Model file for the job. Use its own axes, mm. A direction names the side the tool comes from. Round coordinates to 2 decimals unless told otherwise and drop trailing zeros. Order: outer loops, then holes, each group sorted by start corner. A loop starts at its lowest first (then second) coordinate and runs counter-clockwise, first axis right, second up. Notation, with made-up numbers: M -35.5,76.5 L 2.5,76.5 A31 cw 2.5,109.5 Z; hole C -11.75,23.5 d10. An arc over 180 degrees is marked long. Return JSON: item names as keys, results as strings. Group by question number.
Item 1: Slice it at A-A on z = 2. Give the number of separate pieces and of enclosed holes in the cut face, then the cut area to 3 significant figures.
Item 2: Which spindle directions (+Z, -Z, +X, -X, +Y, -Y) get a long thin tool onto all of the face, cutting with end or side? Do faces 4 (the face through (-17, 3, 2)), 5 (the face through (-6.25, -6, 0)), 6 (the face through (0, 12, 1)), 7 (the face through (-0.1, -9.2, -2)), 8 (the face through (11, -1, 4)). Say none if no direction does.
Item 3: Slice it at B-B on z = -0.5. Write the cut outline in (x, y) (3 decimals), then the cut area to 3 significant figures.
Item 4: Pin check, flat tips, straight feed: pin 1 Ø1.6 at (x, z) = (-17, 1.5) entering from +Y; pin 2 Ø2.5 at (x, y) = (-12, 0) entering from +Z; pin 3 Ø5 at (x, z) = (-3, 0) entering from +Y; pin 4 Ø2.5 at (x, y) = (0, 16) entering from -Z. Stop position of each tip, or through.
Item 5: Probe line 1 along Y through (x, z) = (0, 2) (3 decimals); line 2 along X through (y, z) = (14, 3.25); line 3 along X through (y, z) = (3, 4.5). List the from-to ranges inside material, lowest first.
Item 6: Pull direction X, two halves, no side cores. Call faces 1 (the face through (17, 3, 2)), 2 (the face through (0, 18, 2)), 3 (the face through (-8, -8, 1)): pulls with the +X half, pulls with the -X half, needs draft (parallel to the pull), parting line crosses it, or undercut.
Autodesk Inventor part; units mm, degrees
ref_plane "YZ Plane" through (0, 0, 0) normal (1, 0, 0) x (0, 1, 0)
ref_plane "XZ Plane" through (0, 0, 0) normal (0, 1, 0) x (-1, 0, 0)
ref_plane "XY Plane" through (0, 0, 0) normal (0, 0, 1) x (1, 0, 0)
sketch "Sketch1" plane through (0, 0, 0) normal (0, 0, 1) x (1, 0, 0)
  circle A0 centre (0, 0) radius 18
  line L0 (0, 0) -> (0, 18) construction
  line L1 (4, 17.5499) -> (4, 11.9999)
  line L2 (4, 11.9999) -> (8.5659, 15.8312)
  line L3 (0, 0) -> (18, 0) construction
  line L4 (-4, 17.5499) -> (-4, 11.9999)
  line L5 (-4, 11.9999) -> (-8.5659, 15.8312)
  line L6 (4, -17.5499) -> (4, -11.9999)
  line L7 (4, -11.9999) -> (8.5659, -15.8312)
  line L8 (-4, -11.9999) -> (-8.5659, -15.8312)
  line L9 (-4, -17.5499) -> (-4, -11.9999)
  dimension "d1" = 50
  dimension "d2" = 36
  dimension "d3" = 5.55
  dimension "d4" = 8
extrude "Extrusion1" add sketch "Sketch1" along normal blind 3.5
sketch "Sketch2" plane through (0, 0, 0) normal (0, 1, 0) x (-1, 0, 0)
  line L0 (0, 0) -> (0, 6)
  line L1 (0, 6) -> (-3.5, 6)
  line L2 (-3.5, 6) -> (-6.875, 3.5)
  line L3 (8.5659, 3.5) -> (-18, 3.5)
  line L4 (8.5659, 0) -> (8.5659, 0)
  line L5 (-6.875, 3.5) -> (0, 3.5)
  line L6 (-8.5659, 3.5) -> (-4, 3.5)
  point P0 (-18, 0)
  point P1 (18, 0)
  dimension "d7" = 3.5
  dimension "d8" = 6
  dimension "d9" = 13.75
revolve "Revolution1" add sketch "Sketch2" angle 360 about axis through (0, 0, 0) along (0, 0, 1)
sketch "Sketch6" plane through (0, 0, 0) normal (1, 0, 0) x (0, 1, 0)
  circle A0 centre (-18, 0.2) radius 0.2
  line L0 (18, 0) -> (-18, 0)
  line L1 (-18, 0) -> (-18, 3.5)
  line L2 (0, 0) -> (0, 9.8131)
  point P0 (-18, 0.4)
  dimension "d28" = 0.4
revolve "Revolution2" add sketch "Sketch6" angle 360 about axis through (0, 0, 0) along (0, 0, 1) picked at (-18.0623, 0.1764) contours A0 L1
sketch "Sketch7" plane through (0, 0, 3.5) normal (0, 0, 1) x (1, 0, 0)
  line L0 (4, 17.5499) -> (4, 11.9999)
  line L1 (4, 11.9999) -> (8.5659, 15.8312)
  line L2 (-4, 17.5499) -> (-4, 11.9999)
  line L3 (-4, 11.9999) -> (-8.5659, 15.8312)
  line L4 (-4, -11.9999) -> (-8.5659, -15.8312)
  line L5 (-4, -17.5499) -> (-4, -11.9999)
  line L6 (4, -17.5499) -> (4, -11.9999)
  line L7 (4, -11.9999) -> (8.5659, -15.8312)
  line L8 (4, -17.5499) -> (4, -18.3914)
  line L9 (8.5659, -15.8312) -> (9.2402, -16.397)
  line L10 (0, 0) -> (0, -19.1276)
  line L11 (0, 0) -> (-12.703, 0)
  circle A0 centre (0, 0) radius 18.8214
  line L12 (-4, -17.5499) -> (-4, -18.3914)
  line L13 (-8.5659, -15.8312) -> (-9.2402, -16.397)
  line L14 (4, 17.5499) -> (4, 18.3914)
  line L15 (8.5659, 15.8312) -> (9.2402, 16.397)
  line L16 (-4, 17.5499) -> (-4, 18.3914)
  line L17 (-8.5659, 15.8312) -> (-9.2402, 16.397)
extrude "Extrusion5" cut sketch "Sketch7" against normal through all contours L14 A0 L15 L1 L0 | L16 L2 L3 L17 A0 | A0 L8 L6 L7 L9 | L13 L4 L5 L12 A0
sketch "Sketch4" plane through (0, 0, 3.5) normal (0, 0, 1) x (1, 0, 0)
  line L0 (0, 0) -> (0, -18)
  arc A0 (-8.5659, 15.8312) -> (-8.5659, -15.8312) centre (0, 0) ccw
  line L1 (0, -8.925) -> (-6.25, -8.925)
  line L2 (-6.25, -8.925) -> (-6.25, -6.875)
  line L3 (-6.25, -6.875) -> (0, -6.875)
  circle A1 centre (0, 0) radius 6.875
  line L4 (0, -8.925) -> (6.25, -8.925)
  line L5 (6.25, -8.925) -> (6.25, -6.875)
  line L6 (6.25, -6.875) -> (0, -6.875)
  point P0 (-4, -17.5499)
  point P1 (4, -17.5499)
  dimension "d12" = 2.05
  dimension "d13" = 12.5
extrude "Extrusion2" cut sketch "Sketch4" against normal through all contours L6 L5 L4 L0 | L0 L1 L2 L3
sketch "Sketch3" plane through (0, 0, 0) normal (0, 0, -1) x (-1, 0, 0)
  line L0 (8.5659, -15.8312) -> (4, -11.9999)
  line L1 (8.5659, -15.8312) -> (4, -11.9999)
  line L2 (4, -11.9999) -> (8, -11.9999)
  line L3 (8, -11.9999) -> (8, -3.9)
  line L4 (8, -3.9) -> (-1.347, -3.9)
  line L5 (0, 0) -> (0, -22.6953) construction
  line L6 (8.5659, -15.8312) -> (9.347, -21.3508)
  line L7 (9.347, -21.3508) -> (0, -21.3508)
  line L8 (4, 11.9999) -> (8.5659, 15.8312)
  line L9 (8.5659, 15.8312) -> (4, 11.9999)
  line L10 (4, 11.9999) -> (-4, 11.9999)
  line L11 (-8.5659, 15.8312) -> (-4, 11.9999)
  line L12 (-4, 11.9999) -> (-8.5659, 15.8312)
  line L13 (-8.5659, 15.8312) -> (-8.5659, 22.0204)
  line L14 (-8.5659, 22.0204) -> (9.347, 21.5839)
  line L15 (9.347, 21.5839) -> (8.5659, 15.8312)
  line L16 (-8.5659, -15.8312) -> (-4, -11.9999)
  line L17 (-4, -11.9999) -> (-8, -11.9999)
  line L18 (-8, -11.9999) -> (-8, -3.9)
  line L19 (-8, -3.9) -> (-1.347, -3.9)
  line L20 (-8.5659, -15.8312) -> (-9.347, -21.3508)
  line L21 (-9.347, -21.3508) -> (0, -21.3508)
  line L22 (6.25, -8.925) -> (6.25, -6.875)
  line L23 (6.25, -7.9) -> (0, -7.9) construction
  line L24 (6.25, -7.9) -> (6.25, -5.4)
  line L25 (6.25, -5.4) -> (6.25, -3.9)
  dimension "d11" = 16
  dimension "d16" = 2.5
  dimension "d17" = 1.5
extrude "Extrusion3" cut sketch "Sketch3" against normal blind 1.5
sketch "Sketch5" plane through (0, 0, 0) normal (1, 0, 0) x (0, 1, 0)
  line L0 (-6.875, 1.5) -> (-8.925, 1.5)
  line L1 (-6.875, 1.5) -> (-6.875, -2.7432)
  line L2 (-11.9999, 1.5) -> (-3.9, 1.5)
  line L3 (-5.45, 1.5) -> (-5.7054, -2.1568)
  line L4 (-7.95, 1.5) -> (-7.95, -5) construction
  circle A0 centre (-7.95, -2) radius 1.25
  circle A1 centre (-7.95, -5) radius 2.5
  circle A2 centre (-7.95, -2) radius 2.25
  line L5 (-10.45, 1.5) -> (-10.1945, -2.1568)
  line L6 (-6.875, 3.5) -> (-8.925, 3.5)
  line L7 (-8.925, 3.5) -> (-8.925, 1.5)
  line L8 (-8.925, 1.5) -> (-8.925, -1.2178)
  line L9 (-8.925, 0.0278) -> (-8.925, -1.2178)
  line L10 (-5.45, 1.5) -> (-5.45, 0) construction
  line L11 (-11.9999, 0) -> (-3.9, 0)
  point P0 (0, 0)
  point P1 (-9.0249, -0.0234)
  point P2 (-6.875, -1.3621)
  point P3 (-6.9273, -2.7187)
  point P4 (-6.115, -3.3021)
  point P5 (-9.7849, -3.3021)
  point P6 (-8.9727, -2.7188)
  point P7 (-6.875, -2.6379)
  point P8 (-6.875, -2.7429)
  dimension "d21" = 2.5
  dimension "d20" = 5
  dimension "d22" = 4.5
  dimension "d23" = 5
  dimension "d24" = 5.5
  dimension "d25" = 3
extrude "Extrusion4" add sketch "Sketch5" along normal mid plane 12.5 contours L2 L3 L11 L1 | L8 A2 L11 L5 L2 | L11 L3 A2 L1 | L8 L11 A2 | A2 A1 L1 A0 | L11 A2 L5 | L11 L8 A0 A1 A2 | L1 A1 A0 picked at (-8.956, 0.0031) picked at (-6.8805, -2.682)
sketch "Sketch9" plane through (0, 0, 3.5) normal (0, 0, 1) x (1, 0, 0)
  line L0 (0, 0) -> (0, 19.9091)
  line L1 (0, 0) -> (-25.5758, 0)
  line L2 (-20.3636, 0) -> (-20.3636, 3)
  line L3 (-20.3636, 3) -> (-16.5, 3)
  line L4 (-16.5, 3) -> (-16.5, 0)
  line L5 (-20.3636, 0) -> (-20.3636, -3)
  line L6 (-16.5, -3) -> (-16.5, 0)
  line L7 (-20.3636, -3) -> (-16.5, -3)
  line L8 (20.3636, 0) -> (20.3636, 3)
  line L9 (20.3636, 3) -> (16.5, 3)
  line L10 (16.5, 3) -> (16.5, 0)
  line L11 (20.3636, 0) -> (20.3636, -3)
  line L12 (16.5, -3) -> (16.5, 0)
  line L13 (20.3636, -3) -> (16.5, -3)
  dimension "d34" = 6
  dimension "d35" = 33
extrude "Extrusion6" cut sketch "Sketch9" against normal through all
sketch "Sketch10" plane through (0, 0, 3.5) normal (0, 0, 1) x (1, 0, 0)
  circle A0 centre (-12.5, 0) radius 4
  line L0 (-12.5, 3.2505) -> (-9.685, 1.6252)
  line L1 (-9.685, 1.6252) -> (-9.685, -1.6252)
  line L2 (-9.685, -1.6252) -> (-12.5, -3.2505)
  line L3 (-12.5, -3.2505) -> (-15.315, -1.6252)
  line L4 (-15.315, -1.6252) -> (-15.315, 1.6252)
  line L5 (-15.315, 1.6252) -> (-12.5, 3.2505)
  line L6 (-12.5, 0) -> (-12.5, 3.2505)
  line L7 (-16.5, 3) -> (-16.5, -3)
  line L8 (0, 0) -> (0, 18.074)
  circle A1 centre (12.5, 0) radius 4
  line L9 (12.5, 3.2505) -> (9.685, 1.6252)
  line L10 (9.685, 1.6252) -> (9.685, -1.6252)
  line L11 (9.685, -1.6252) -> (12.5, -3.2505)
  line L12 (12.5, -3.2505) -> (15.315, -1.6252)
  line L13 (15.315, -1.6252) -> (15.315, 1.6252)
  line L14 (15.315, 1.6252) -> (12.5, 3.2505)
  line L15 (12.5, 0) -> (12.5, 3.2505)
  dimension "d38" = 8
  dimension "d42" = 5.63
extrude "Extrusion7" add sketch "Sketch10" along normal blind 5 from surface at -3.5
sketch "Sketch11" plane through (0, 0, 3.5) normal (0, 0, 1) x (1, 0, 0)
  circle A0 centre (-12.5, 0) radius 4
  circle A1 centre (-12.5, 0) radius 1.25
  circle A2 centre (0, 16) radius 1.5
  circle A3 centre (-9.5, 7.5) radius 2.75
  line L0 (0, 0) -> (0, 18) construction
  arc A4 (4, 17.5499) -> (-4, 17.5499) centre (0, 0) ccw
  line L1 (0, 0) -> (6.926, 0) construction
  circle A5 centre (0, -16) radius 1.5
  circle A6 centre (12.5, 0) radius 1.25
  circle A7 centre (9.5, 7.5) radius 2.75
  point P0 (-16.5, 0)
  dimension "d43" = 2.5
  dimension "d44" = 3
  dimension "d45" = 5.5
  dimension "d46" = 7.5
  dimension "d47" = 19
  dimension "d48" = 32
extrude "Extrusion8" cut sketch "Sketch11" against normal through all contours A1 | A2 | A3 | A5 | A6 | A7
sketch "Sketch12" plane through (0, 0, 0) normal (0, 0, -1) x (-1, 0, 0)
  circle A0 centre (0, 0) radius 2
  dimension "d54" = 4
extrude "Extrusion9" cut sketch "Sketch12" against normal blind 3.5
sketch "Sketch13" plane through (0, 0, 3.5) normal (0, 0, 1) x (1, 0, 0)
  circle A0 centre (12.5, 0) radius 1.25
  line L0 (12.5, 3.2505) -> (9.685, 1.6252)
  line L1 (9.685, 1.6252) -> (9.685, -1.6252)
  line L2 (9.685, -1.6252) -> (12.5, -3.2505)
  line L3 (12.5, -3.2505) -> (15.315, -1.6252)
  line L4 (15.315, -1.6252) -> (15.315, 1.6252)
  line L5 (15.315, 1.6252) -> (12.5, 3.2505)
  circle A1 centre (-12.5, 0) radius 1.25
  line L6 (-12.5, 3.2505) -> (-15.315, 1.6252)
  line L7 (-15.315, 1.6252) -> (-15.315, -1.6252)
  line L8 (-15.315, -1.6252) -> (-12.5, -3.2505)
  line L9 (-12.5, -3.2505) -> (-9.685, -1.6252)
  line L10 (-9.685, -1.6252) -> (-9.685, 1.6252)
  line L11 (-9.685, 1.6252) -> (-12.5, 3.2505)
  point P0 (0, 0)
extrude "Extrusion10" add sketch "Sketch13" along normal blind 0.5
chamfer "Chamfer2" distance 0.3 angle 45 6 edges at (11.25, 0, 4) (-13.75, 0, 4) (-1.5, -16, 3.5) (-1.5, 16, 3.5) (-13.75, 0, 0) (11.25, 0, 0)
properties part number "18102021-002-02" material "Stainless Steel"
Output values:
{
 "1": {"separate pieces": "1", "enclosed holes": "8", "area": "838 mm²"},
 "2": {"face 4": "+Z, -Z, -X", "face 5": "-Z", "face 6": "-Z, +Y", "face 7": "+X, -X", "face 8": "+Z"},
 "3": {"outline": "M -6.25,-10.31 L 6.25,-10.31 L 6.25,-8.925 L -6.25,-8.925 Z; M -6.25,-6.875 L 6.25,-6.875 L 6.25,-5.59 L -6.25,-5.59 Z", "area": "33.4 mm²"},
 "4": {"pin 1": "y = 7.85", "pin 2": "z = 4", "pin 3": "y = 17.97", "pin 4": "through"},
 "5": {"line 1": "-18 to -17.5, -14.5 to -8.925, -6.875 to -2, 2 to 14.5, 17.5 to 18", "line 2": "-11.31 to -6.38, -4 to 4, 6.38 to 11.31", "line 3": "-15.15 to -12.93, -12.07 to -9.85, -4.64 to 4.64, 9.85 to 12.07, 12.93 to 15.15"},
 "6": {"face 1": "needs draft", "face 2": "parting line crosses it", "face 3": "undercut"}
}
